Can you work these out from the model? Positions are in its coordinate system, mm. Face numbers are marked on the shaded views. A direction names the side the tool comes from. Round coordinates to 2 decimals unless told otherwise and drop trailing zeros. Order: outer loops, then holes, each group sorted by start corner. A loop starts at its lowest first (then second) coordinate and runs counter-clockwise, first axis right, second up. Notation, with made-up numbers: M 74.5,26.25 L 95.5,26.25 A9 ccw 95.5,30.25 Z; hole C -11.75,15 d6. An arc over 180 degrees is marked long. One line per question, with ' | ' between items.
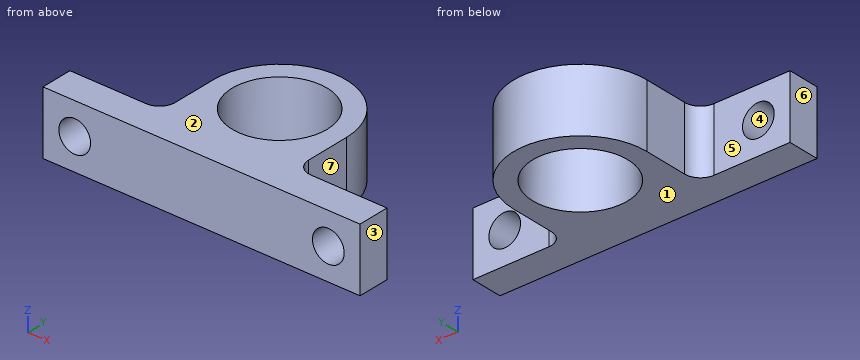
```python
from build123d import *

# Parameters (mm, degrees)
SKETCH1_R           = 7.5
BOSS_EXTRUDE1_DEPTH = 10
SKETCH3_R           = 2.5
CUT_EXTRUDE1_DEPTH  = 22


with BuildPart() as part:
    # Sketch1 → Boss-Extrude1 (new body)
    with BuildSketch(Plane.XY):
        with BuildLine():
            Line((25, 0), (-25, 0))
            Line((-25, 0), (-25, 5))
            Line((-25, 5), (-13, 5))
            ThreePointArc((-13, 5), (-11.232233047, 5.732233047), (-10.5, 7.5))
            Line((-10.5, 7.5), (-10.5, 14.5))
            ThreePointArc((-10.5, 14.5), (0, 25), (10.5, 14.5))
            Line((10.5, 14.5), (10.5, 7.5))
            ThreePointArc((10.5, 7.5), (11.232233047, 5.732233047), (13, 5))
            Line((13, 5), (25, 5))
            Line((25, 5), (25, 0))
        make_face()
        with Locations((0, 14.5)):
            Circle(SKETCH1_R, mode=Mode.SUBTRACT)
    extrude(amount=BOSS_EXTRUDE1_DEPTH)

    # Sketch3 → Cut-Extrude1 (cut)
    with BuildSketch(Plane(origin=(0, 5, 0), x_dir=(1, 0, 0), z_dir=(0, 1, 0))):
        with Locations(Location((-20, -5, 0), (0, 0, 270))):
            Circle(SKETCH3_R)
        with Locations(Location((20, -5, 0), (0, 0, 270))):
            Circle(SKETCH3_R)
    extrude(amount=-CUT_EXTRUDE1_DEPTH, mode=Mode.SUBTRACT)


solid = part.part
```
(1) If we section it at B-B on y = 9.75: Please give me the cut outline in (x, z).
Final values:
outline: M -10.5,0 L -5.8,0 L -5.8,10 L -10.5,10 Z; M 5.8,0 L 10.5,0 L 10.5,10 L 5.8,10 Z
(2) If we section it at C-C on z = 9: Please give me the cut outline in (x, y), plus the area to 3 significant figures.
Final values:
outline: M -25,0 L 25,0 L 25,5 L 13,5 A2.5 cw 10.5,7.5 L 10.5,14.5 A10.5 ccw -10.5,14.5 L -10.5,7.5 A2.5 cw -13,5 L -25,5 Z; hole C 0,14.5 d15 | area: 449 mm^2
(3) On a 3-axis mill with a long thin cutter (end or side, diameter ignored), from which of +Z, -Z, +X, -X, +Y, -Y can I reach the whole of each face in a straight line? I mean the marked faces 5, 6 and 7. Say none if no direction works.
Final values:
face 5: +Z, -Z, -X, +Y | face 6: +Z, -Z, -X, +Y, -Y | face 7: +Z, -Z, +X, +Y
(4) Will these pins go through, and if not, where does the flat tip stop? pin 1 Ø3 at (y, z) = (11, 6.5) entering from -X; pin 2 Ø2 at (y, z) = (12.5, 5.5) entering from +X; pin 3 Ø4 at (x, y) = (-1.5, 8.5) entering from -Z; pin 4 Ø3 at (x, z) = (-19, 7) entering from +Y.
Final values:
pin 1: x = -10.5 | pin 2: x = 10.5 | pin 3: z = 0 | pin 4: y = 5
(5) If we section it at A-A on x = 18: Please give me the cut outline in (y, z).
Final values:
outline: M 0,0 L 5,0 L 5,3.5 L 0,3.5 Z; M 0,6.5 L 5,6.5 L 5,10 L 0,10 Z
(6) If we section it at D-D on y = 2.25: Please give me the cut outline in (x, z).
Final values:
outline: M -25,0 L 25,0 L 25,10 L -25,10 Z; hole C -20,5 d5; hole C 20,5 d5
(7) Thinking about a two-plate mould opening in Z: for the marked faces 1, 2, 3 and 4, which applies, released by +Z, released by -Z, zero draft, split by the parting line, or undercut?
Final values:
face 1: released by -Z | face 2: released by +Z | face 3: zero draft | face 4: undercut
(8) Please list where these lines run through material, in increasing order: probe 1 along X at (y, z) = (3.2, 5); probe 2 along X at (y, z) = (14.25, 2.5); probe 3 along X at (y, z) = (2.25, 7). Write a range as [from, to].
Final values:
probe 1: [-25, -22.5], [-17.5, 17.5], [22.5, 25] | probe 2: [-10.5, -7.5], [7.5, 10.5] | probe 3: [-25, -21.5], [-18.5, 18.5], [21.5, 25]
